```python
from build123d import *

# Parameters (mm, degrees)
F0_R     = 50
F1_DEPTH = 120
F2_T     = -5
F3_R     = 5
F4_R     = 2


with BuildPart() as f1:
    # F0 (on Top) → F1 (new body)
    with BuildSketch(Plane.XY):
        Circle(F0_R)
    extrude(amount=F1_DEPTH)

    # F2
    f2_openings = [f1.faces().sort_by_distance(p)[0] for p in [
        (0, 0, 120),
    ]]
    offset(amount=F2_T, openings=f2_openings)

    # F3
    f3_edges = [f1.edges().sort_by_distance(p)[0] for p in [
        (-45, 0, 5),
        (-50, 0, 0),
    ]]
    fillet(f3_edges, radius=F3_R)

    # F4
    f4_edges = [f1.edges().sort_by_distance(p)[0] for p in [
        (-45, 0, 120),
        (-50, 0, 120),
    ]]
    fillet(f4_edges, radius=F4_R)


solid = f1.part
```
Work out the finished part from the listing and answer in its coordinate system (mm). A direction names the side the tool comes from. Round coordinates to 2 decimals unless told otherwise and drop trailing zeros. Write each loop counter-clockwise with the first axis right and the second up, starting at its lowest first coordinate (ties: lowest second). Pieces come first, ordered by that corner, then holes. Notation, with made-up numbers: (-25.5, 22.5) -> (4.5, 22.5) arc R16 ccw to (4.5, 43.5) -> close; hole circle Ø1 at (57.25, -26.75). An arc over 180 degrees is marked (long way). Write each question's results on one line, items separated by ' | '.
1) For a pull along Y with two mould halves and no side action, classify faces 3 (the flat face through (35, -32, 120)), 4 (the cylindrical face through (20.765, -39.923, 63.244)), 5 (the cylindrical face through (47.69, 15.02, 60.71)) as +Y half, -Y half, draft (parallel to the pull), parting line (faces both ways), or undercut.
Findings:
face 3: draft | face 4: undercut | face 5: parting line
2) Flat-ended cylindrical pins translate along their axes: pin 1 (6 mm diameter, centred on x = 4.5, y = -29.5, fed in from -Z); pin 2 (1 mm diameter, centred on y = -13, z = 53, fed in from +X); pin 3 (5 mm diameter, centred on y = 38, z = 87, fed in from +X); pin 4 (24 mm diameter, centred on x = 13.5, y = -9, fed in from +Z). Find the tip coordinate at first contact, or state that the pin passes through.
Findings:
pin 1: stops at z = 0 | pin 2: stops at x = 48.41 | pin 3: stops at x = 35.21 | pin 4: stops at z = 5
3) The part is cut by section A-A (x = 0). Write down the section's boundary in (y, z), and give its area (3 significant figures).
Findings:
outline: (-50, 5) arc R5 ccw to (-45, 0) -> (45, 0) arc R5 ccw to (50, 5) -> (50, 118) arc R2 ccw to (48, 120) -> (47, 120) arc R2 ccw to (45, 118) -> (45, 10) arc R5 cw to (40, 5) -> (-40, 5) arc R5 cw to (-45, 10) -> (-45, 118) arc R2 ccw to (-47, 120) -> (-48, 120) arc R2 ccw to (-50, 118) -> close | area: 1,650 mm²
4) The part is cut by section C-C (z = 87.5). Write down the section's boundary in (x, y), and give its area (3 significant figures).
Findings:
outline: circle Ø100 at (0, 0); hole circle Ø90 at (0, 0) | area: 1,490 mm²
5) Consider line 1 along Y through (x, z) = (0, 50); line 2 along X through (y, z) = (39.5, 29); line 3 along X through (y, z) = (7, 69.5). Determine where each line is inside the solid, lowest interval first. Write a range as [from, to].
Findings:
line 1: y = [-50, -45], [45, 50] | line 2: x = [-30.66, -21.56], [21.56, 30.66] | line 3: x = [-49.51, -44.45], [44.45, 49.51]
6) Which of the six approach directions +Z, -Z, +X, -X, +Y, -Y give full straight-line access (tool end or side, diameter ignored) to faces 1 (the flat face through (-1, 1, 5)), 2 (the flat face through (-1, 1, 0))?
Findings:
face 1: +Z | face 2: -Z, +X, -X, +Y, -Y
